CAD build for the part. Positions are in the model's coordinates, mm. Face numbers are marked on the shaded views. A direction names the side the tool comes from. Round coordinates to 2 decimals unless told otherwise and drop trailing zeros. Loops run counter-clockwise (first coordinate to the right, second up) from the corner with the lowest first, then second, coordinate; pieces in that order, holes last. Notation, with made-up numbers: (6, -33) - (35, -33) arc R11 cw to (35, -18) - close; hole circle Ø9 at (-3.5, 20). An arc over 180 degrees is marked (long way). One line per question, with ' | ' between items.
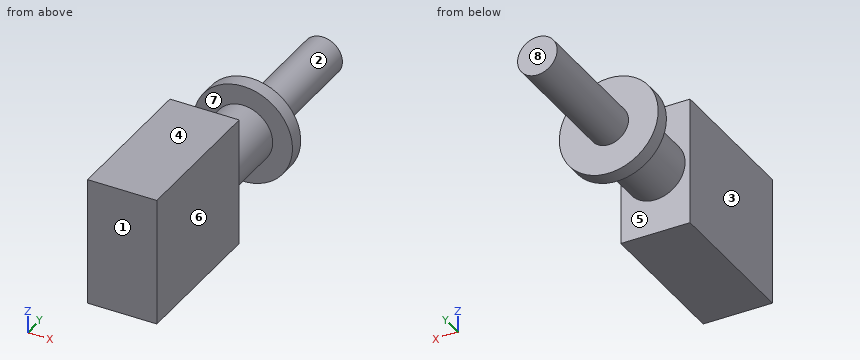
```python
from build123d import *

# Parameters (mm, degrees)
ESQUISSE1_W      = 7
ESQUISSE1_H      = 13
EXTRUSION1_DEPTH = 15
ESQUISSE2_R      = 3
EXTRUSION2_DEPTH = 7
ESQUISSE3_R      = 5
EXTRUSION3_DEPTH = 1.5
ESQUISSE4_R      = 2
EXTRUSION4_DEPTH = 13


with BuildPart() as part:
    # Esquisse1 → Extrusion1 (new body)
    with BuildSketch(Plane(origin=(0, 0, 0), x_dir=(1, 0, 0), z_dir=(0, 1, 0))):
        Rectangle(ESQUISSE1_W, ESQUISSE1_H)
    extrude(amount=EXTRUSION1_DEPTH)

    # Esquisse2 → Extrusion2 (add)
    with BuildSketch(Plane(origin=(0, 15, 0), x_dir=(-1, 0, 0), z_dir=(0, 1, 0))):
        with Locations(Location((0, 0, 0), (0, 0, 270))):
            Circle(ESQUISSE2_R)
    extrude(amount=EXTRUSION2_DEPTH)

    # Esquisse3 → Extrusion3 (add)
    with BuildSketch(Plane(origin=(0, 22, 0), x_dir=(-1, 0, 0), z_dir=(0, 1, 0))):
        with Locations(Location((0, 0, 0), (0, 0, 90))):
            Circle(ESQUISSE3_R)
    extrude(amount=EXTRUSION3_DEPTH)

    # Esquisse4 → Extrusion4 (add)
    with BuildSketch(Plane(origin=(0, 23.5, 0), x_dir=(-1, 0, 0), z_dir=(0, 1, 0))):
        with Locations(Location((0, 0, 0), (0, 0, 270))):
            Circle(ESQUISSE4_R)
    extrude(amount=EXTRUSION4_DEPTH)


solid = part.part
```
(1) Cut at C-C, the plane y = 32.5. Write the cut outline in (x, z), then the cut area to 3 significant figures.
Results found:
outline: circle Ø4 at (0, 0) | area: 12.6 mm²
(2) Cut at A-A, the plane x = 0. Write the cut outline in (y, z), then the cut area to 3 significant figures.
Results found:
outline: (0, -6.5) - (15, -6.5) - (15, -3) - (22, -3) - (22, -5) - (23.5, -5) - (23.5, -2) - (36.5, -2) - (36.5, 2) - (23.5, 2) - (23.5, 5) - (22, 5) - (22, 3) - (15, 3) - (15, 6.5) - (0, 6.5) - close | area: 304 mm²
(3) Tool access for the marked faces 1, 2, 3, 4 and 5: list every direction of +Z, -Z, +X, -X, +Y, -Y with a clear straight run to the whole face (end or side of a thin tool).
Results found:
face 1: +Z, -Z, +X, -X, -Y | face 2: +Y | face 3: +Z, -Z, -X, -Y | face 4: +Z, +X, -X, +Y, -Y | face 5: none
(4) Two-plate mould, pull along Y, no slides. Class the marked faces 6, 7 and 8: released by +Y, released by -Y, zero draft, split by the parting line, or undercut.
Results found:
face 6: zero draft | face 7: undercut | face 8: released by +Y
(5) Cut at B-B, the plane z = 0. Write the cut outline in (x, y).
Results found:
outline: (-5, 22) - (-3, 22) - (-3, 15) - (-3.5, 15) - (-3.5, 0) - (3.5, 0) - (3.5, 15) - (3, 15) - (3, 22) - (5, 22) - (5, 23.5) - (2, 23.5) - (2, 36.5) - (-2, 36.5) - (-2, 23.5) - (-5, 23.5) - close
(6) Cut at D-D, the plane y = 9. Write the cut outline in (x, z), then the cut area to 3 significant figures.
Results found:
outline: (-3.5, -6.5) - (3.5, -6.5) - (3.5, 6.5) - (-3.5, 6.5) - close | area: 91.0 mm²
(7) Drop flat-ended pins along their axis: P1, Ø3, axis at y = 26, z = -2.5, coming from the -X side; P2, Ø2, axis at x = -2, y = 22, coming from the +Z side. Give the stop position or say it passes through.
Results found:
P1: stops at x = -1.73 | P2: stops at z = 4.9
(8) Probe L1, parallel to Y at x = -3.25, z = 1.5; L2, parallel to Y at x = -3, z = 4.5; L3, parallel to X at y = 5, z = 6.25. List the from-to ranges inside material, lowest first.
Results found:
L1: y = 0 to 15, 22 to 23.5 | L2: y = 0 to 15 | L3: x = -3.5 to 3.5
